from build123d import *

# Parameters (mm, degrees)
EXTRUDE_1_DEPTH                  = 35
SKETCH_2_W                       = 22
SKETCH_2_H                       = 35
EXTRUDE_2_DEPTH                  = 22.75
SKETCH_3_W                       = 11
SKETCH_3_H                       = 15
CUT_EXTRUDE_1_DEPTH              = 32
HOLE_WIZARD_12_5_12_5_1_D        = 12.5
HOLE_WIZARD_12_5_12_5_2_D        = 12.5
HOLE_WIZARD_3_5_3_5_1_D          = 3.5
HOLE_WIZARD_3_5_3_5_1_DEPTH      = 5
SKETCH_10_W                      = 9.5
SKETCH_10_H                      = 18.75
CUT_EXTRUDE_2_DEPTH              = 64.639610362
SKETCH_11_W                      = 22.75
SKETCH_11_H                      = 11
CUT_EXTRUDE_3_DEPTH              = 15
FILLET_2_R                       = 10
SKETCH_13_W                      = 4
SKETCH_13_H                      = 30
EXTRUDE_3_DEPTH                  = 31
SKETCH_16_W                      = 1.75
SKETCH_16_H                      = 4
HOLE_WIZARD_3_5_3_5_2_AT_2_COUNT = 2
HOLE_WIZARD_3_5_3_5_2_AT_2_PITCH = 24
HOLE_WIZARD_3_5_3_5_2_AT_3_COUNT = 2
HOLE_WIZARD_3_5_3_5_2_AT_3_PITCH = 33.941125497
HOLE_WIZARD_3_5_3_5_2_AT_4_COUNT = 2
HOLE_WIZARD_3_5_3_5_2_AT_4_PITCH = 24
SKETCH_17_R                      = 14
CUT_EXTRUDE_4_DEPTH              = 76.494728698
SKETCH_19_W                      = 4
SKETCH_19_H                      = 30
EXTRUDE_5_DEPTH                  = 34
SKETCH_20_R                      = 14
CUT_EXTRUDE_5_DEPTH              = 76.494728698
SKETCH_22_W                      = 1.75
SKETCH_22_H                      = 4
HOLE_WIZARD_3_5_3_5_3_AT_2_COUNT = 2
HOLE_WIZARD_3_5_3_5_3_AT_2_PITCH = 24
HOLE_WIZARD_3_5_3_5_3_AT_3_COUNT = 2
HOLE_WIZARD_3_5_3_5_3_AT_3_PITCH = 33.941125497
HOLE_WIZARD_3_5_3_5_3_AT_4_COUNT = 2
HOLE_WIZARD_3_5_3_5_3_AT_4_PITCH = 24
EXTRUDE_6_DEPTH                  = 4
EXTRUDE_7_DEPTH                  = 4
SKETCH_26_W                      = 10
SKETCH_26_H                      = 4
EXTRUDE_8_DEPTH                  = 35
HOLE_WIZARD_3_5_3_5_4_D          = 3.5
FILLET_7_R                       = 2
FILLET_9_R                       = 5
FILLET_10_R                      = 10
FILLET_12_R                      = 10
FILLET_13_R                      = 2
FILLET_14_R                      = 2
CUT_EXTRUDE_6_DEPTH              = 86.007352664
CUT_EXTRUDE_7_DEPTH              = 15
FILLET_15_R                      = 10


# Some blends are built 0.0001 mm under size
with BuildPart() as part:
    # Sketch 1 → Extrude 1 (new body)
    with BuildSketch(Plane(origin=(0, 35, 0), x_dir=(1, 0, 0), z_dir=(0, 1, 0))):
        with BuildLine():
            Line((35, 0), (13, 0))
            Line((13, 0), (13, -28))
            ThreePointArc((13, -28), (16.514718626, -36.485281374), (25, -40))
            ThreePointArc((25, -40), (32.16515139, -35.913807126), (35, -28.167840434))
            Line((35, -28.167840434), (35, 0))
        make_face()
    extrude(amount=-EXTRUDE_1_DEPTH)

    # Sketch 2 → Extrude 2 (add)
    with BuildSketch(Plane.ZY.offset(-13)):
        with Locations((11, 17.5)):
            Rectangle(SKETCH_2_W, SKETCH_2_H)
    extrude(amount=EXTRUDE_2_DEPTH)

    # Sketch 3 → Cut-Extrude 1 (cut)
    with BuildSketch(Plane.ZY.offset(9.75)):
        with Locations((5.5, 7.5)):
            Rectangle(SKETCH_3_W, SKETCH_3_H)
    extrude(amount=-CUT_EXTRUDE_1_DEPTH, mode=Mode.SUBTRACT)

    # Hole Wizard 12.5 _12.5_1 (through all)
    with Locations(Plane(origin=(0, 35, 0), x_dir=(1, 0, 0), z_dir=(0, 1, 0))):
        with Locations((24, -29)):
            Hole(HOLE_WIZARD_12_5_12_5_1_D / 2)

    # Hole Wizard 12.5 _12.5_2 (through all)
    with Locations(Plane(origin=(35, 0, 0), x_dir=(0, 0, -1), z_dir=(1, 0, 0))):
        with Locations((-11, 25)):
            Hole(HOLE_WIZARD_12_5_12_5_2_D / 2)

    # Hole Wizard 3.5 _3.5_1
    with Locations(Plane(origin=(0, 15, 0), x_dir=(-1, 0, 0), z_dir=(0, -1, 0))):
        with Locations((-17.25, -7), (6.75, -7), (-12.25, -7), (1.75, -7)):
            Hole(HOLE_WIZARD_3_5_3_5_1_D / 2, depth=HOLE_WIZARD_3_5_3_5_1_DEPTH)

    # Sketch 10 → Cut-Extrude 2 (cut, through all)
    with BuildSketch(Plane.XZ):
        with Locations((30.25, 9.375)):
            Rectangle(SKETCH_10_W, SKETCH_10_H)
    extrude(amount=-CUT_EXTRUDE_2_DEPTH, mode=Mode.SUBTRACT)

    # Sketch 11 → Cut-Extrude 3 (cut)
    with BuildSketch(Plane.XZ):
        with Locations((1.625, 16.5)):
            Rectangle(SKETCH_11_W, SKETCH_11_H)
    extrude(amount=-CUT_EXTRUDE_3_DEPTH, mode=Mode.SUBTRACT)

    # Fillet 2
    fillet_2_edges = [part.edges().sort_by_distance(p)[0] for p in [
        (25, 17.5, 40),
    ]]
    fillet(fillet_2_edges, radius=FILLET_2_R)

    # Sketch 19 → Extrude 5 (add)
    with BuildSketch(Plane.ZY.offset(9.75)):
        with Locations((2, 7.5)):
            Rectangle(SKETCH_19_W, SKETCH_19_H)
    extrude(amount=EXTRUDE_5_DEPTH)

    # Sketch 20 → Cut-Extrude 5 (cut, through all)
    with BuildSketch(Plane.XY.offset(4)):
        with Locations((-28.75, 7.5)):
            Circle(SKETCH_20_R)
    extrude(amount=-CUT_EXTRUDE_5_DEPTH, mode=Mode.SUBTRACT)

    # Sketch 22 → Hole Wizard 3.5 _3.5_3 (revolve, cut)
    with BuildSketch(Plane(origin=(-16.75, 19.5, 4), x_dir=(0, -1, 0), z_dir=(1, 0, 0))):
        with Locations((0.875, 2)):
            Rectangle(SKETCH_22_W, SKETCH_22_H)
    hole_wizard_3_5_3_5_3 = revolve(axis=Axis((-16.75, 19.5, 10.35), (0, 0, -1)), mode=Mode.SUBTRACT)

    # Hole Wizard 3.5 _3.5_3 at 2: Hole Wizard 3.5 _3.5_3 ×2
    with Locations(*[(0, -i * HOLE_WIZARD_3_5_3_5_3_AT_2_PITCH, 0) for i in range(1, HOLE_WIZARD_3_5_3_5_3_AT_2_COUNT)]):
        add(hole_wizard_3_5_3_5_3, mode=Mode.SUBTRACT)

    # Hole Wizard 3.5 _3.5_3 at 3: Hole Wizard 3.5 _3.5_3 ×2
    with Locations(*[Vector(-0.7071067811865475, -0.7071067811865476, 0) * (i * HOLE_WIZARD_3_5_3_5_3_AT_3_PITCH) for i in range(1, HOLE_WIZARD_3_5_3_5_3_AT_3_COUNT)]):
        add(hole_wizard_3_5_3_5_3, mode=Mode.SUBTRACT)

    # Hole Wizard 3.5 _3.5_3 at 4: Hole Wizard 3.5 _3.5_3 ×2
    with Locations(*[(-i * HOLE_WIZARD_3_5_3_5_3_AT_4_PITCH, 0, 0) for i in range(1, HOLE_WIZARD_3_5_3_5_3_AT_4_COUNT)]):
        add(hole_wizard_3_5_3_5_3, mode=Mode.SUBTRACT)

    # Sketch 24 → Extrude 6 (add)
    with BuildSketch(Plane.XY.offset(4)):
        Polygon((-9.75, 30.5), (-17.75, 22.5), (-9.75, 22.5), align=None)
    extrude(amount=-EXTRUDE_6_DEPTH)



with BuildPart() as body_2:
    # Sketch 13 → Extrude 3 (new body)
    with BuildSketch(Plane(origin=(25.5, 0, 0), x_dir=(0, 0, -1), z_dir=(1, 0, 0))):
        with Locations((-2, 7.5)):
            Rectangle(SKETCH_13_W, SKETCH_13_H)
    extrude(amount=EXTRUDE_3_DEPTH)

    # Sketch 16 → Hole Wizard 3.5 _3.5_2 (revolve, cut)
    with BuildSketch(Plane(origin=(29.5, -4.5, 4), x_dir=(0, -1, 0), z_dir=(1, 0, 0))):
        with Locations((0.875, 2)):
            Rectangle(SKETCH_16_W, SKETCH_16_H)
    hole_wizard_3_5_3_5_2 = revolve(axis=Axis((29.5, -4.5, 10.35), (0, 0, -1)), mode=Mode.SUBTRACT)

    # Hole Wizard 3.5 _3.5_2 at 2: Hole Wizard 3.5 _3.5_2 ×2
    with Locations(*[(0, i * HOLE_WIZARD_3_5_3_5_2_AT_2_PITCH, 0) for i in range(1, HOLE_WIZARD_3_5_3_5_2_AT_2_COUNT)]):
        add(hole_wizard_3_5_3_5_2, mode=Mode.SUBTRACT)

    # Hole Wizard 3.5 _3.5_2 at 3: Hole Wizard 3.5 _3.5_2 ×2
    with Locations(*[Vector(0.7071067811865475, 0.7071067811865476, 0) * (i * HOLE_WIZARD_3_5_3_5_2_AT_3_PITCH) for i in range(1, HOLE_WIZARD_3_5_3_5_2_AT_3_COUNT)]):
        add(hole_wizard_3_5_3_5_2, mode=Mode.SUBTRACT)

    # Hole Wizard 3.5 _3.5_2 at 4: Hole Wizard 3.5 _3.5_2 ×2
    with Locations(*[(i * HOLE_WIZARD_3_5_3_5_2_AT_4_PITCH, 0, 0) for i in range(1, HOLE_WIZARD_3_5_3_5_2_AT_4_COUNT)]):
        add(hole_wizard_3_5_3_5_2, mode=Mode.SUBTRACT)

    # Sketch 17 → Cut-Extrude 4 (cut, through all)
    with BuildSketch(Plane.XY.offset(4)):
        with Locations((41.5, 7.5)):
            Circle(SKETCH_17_R)
    extrude(amount=-CUT_EXTRUDE_4_DEPTH, mode=Mode.SUBTRACT)


with BuildPart() as part_1:
    add(part.part)

    add(body_2.part)  # Extrude 7 merges body 2
    # Sketch 25 → Extrude 7 (add)
    with BuildSketch(Plane.XY.offset(4)):
        Polygon((33.5, 22.5), (25.5, 30.5), (25.5, 22.5), align=None)
    extrude(amount=-EXTRUDE_7_DEPTH)

    # Sketch 26 → Extrude 8 (add)
    with BuildSketch(Plane.XY.offset(22)):
        with Locations((5.25, 17)):
            Rectangle(SKETCH_26_W, SKETCH_26_H)
    extrude(amount=EXTRUDE_8_DEPTH)

    # Hole Wizard 3.5 _3.5_4 (through all)
    with Locations(Plane(origin=(0, 15, 0), x_dir=(-1, 0, 0), z_dir=(0, -1, 0))):
        with Locations((-5.25, -52), (-5.25, -42), (-5.25, -32)):
            Hole(HOLE_WIZARD_3_5_3_5_4_D / 2)

    # Fillet 7
    fillet_7_edges = [part_1.edges().sort_by_distance(p)[0] for p in [
        (0.25, 17, 22),
        (10.25, 17, 22),
    ]]
    fillet(fillet_7_edges, radius=FILLET_7_R)

    # Fillet 9
    fillet_9_edges = [part_1.edges().sort_by_distance(p)[0] for p in [
        (0.25, 17, 57),
        (10.25, 17, 57),
    ]]
    fillet(fillet_9_edges, radius=FILLET_9_R - 0.0001)  # a hair under: the kernel refuses the full size

    # Fillet 10
    # the kernel refuses this fillet: 10 mm, written as the material it takes off along each edge
    with BuildSketch(Plane(origin=(35, -32.046488893, 18.75), x_dir=(-0.03816406367220006, 0, 0.999271486756239), z_dir=(0, 1, 0))) as fillet_10_piece_1:
        with BuildLine():
            CenterArc((10.360556073, -9.693195649), FILLET_10_R, 75.770650452, 103.082689776)
            Line((0.362558605, -9.493079124), (-0.637241142, -9.473067472))
            ThreePointArc((-0.637241142, -9.473067472), (-0.817992184, -4.784703626), (-0.999271487, -0.038164064))
            Line((-0.999271487, -0.038164064), (-0.038164064, 0.999271487))
            ThreePointArc((-0.038164064, 0.999271487), (9.372815349, 1.358694549), (13.064399506, 0.969319565))
            Line((13.064399506, 0.969319565), (12.818595557, 0))
        make_face()
    extrude(amount=99.092977786, mode=Mode.SUBTRACT)

    # Fillet 12
    fillet_12_edges = [part_1.edges().sort_by_distance(p)[0] for p in [
        (1.625, 35, 22),
    ]]
    fillet(fillet_12_edges, radius=FILLET_12_R)

    # Fillet 13
    fillet_13_edges = [part_1.edges().sort_by_distance(p)[0] for p in [
        (-9.75, 30.5, 2),
        (-9.75, -7.5, 2),
        (-43.75, 22.5, 2),
        (-43.75, -7.5, 2),
        (-17.75, 22.5, 2),
    ]]
    fillet(fillet_13_edges, radius=FILLET_13_R)

    # Fillet 14
    fillet_14_edges = [part_1.edges().sort_by_distance(p)[0] for p in [
        (56.5, 22.5, 2),
        (25.5, 30.5, 2),
        (33.5, 22.5, 2),
        (25.5, -7.5, 2),
        (56.5, -7.5, 2),
    ]]
    fillet(fillet_14_edges, radius=FILLET_14_R)

    # Sketch 32 → Cut-Extrude 6 (cut, through all)
    with BuildSketch(Plane.XY.offset(4)):
        with BuildLine():
            Line((-9.75, 2.270340952), (-9.75, 15))
            ThreePointArc((-9.75, 15), (-10.952290213, 8.635170476), (-9.75, 2.270340952))
        make_face()
    extrude(amount=-CUT_EXTRUDE_6_DEPTH, mode=Mode.SUBTRACT)

    # Sketch 33 → Cut-Extrude 7 (cut)
    with BuildSketch(Plane.XZ):
        with BuildLine():
            Line((13, 22), (13, 11))
            Line((13, 11), (22.25, 11))
            ThreePointArc((22.25, 11), (19.219835157, 17.841111382), (13, 22))
        make_face()
    extrude(amount=-CUT_EXTRUDE_7_DEPTH, mode=Mode.SUBTRACT)

    # Fillet 15
    fillet_15_edges = [part_1.edges().sort_by_distance(p)[0] for p in [
        (13, 7.5, 22),
    ]]
    fillet(fillet_15_edges, radius=FILLET_15_R)


solid = part_1.part
Can you work these out from the model? Positions are in its coordinate system, mm. A direction names the side the tool comes from. Round coordinates to 2 decimals unless told otherwise and drop trailing zeros. Write each loop counter-clockwise with the first axis right and the second up, starting at its lowest first coordinate (ties: lowest second). Pieces come first, ordered by that corner, then holes. Notation, with made-up numbers: M 20,-13.5 L 44,-13.5 A13 cw 44,-6.5 Z; hole C 86.5,34 d8. An arc over 180 degrees is marked long. Use a Markdown table: item, result.
Item 1: I want a section at A-A (z = 42). List the corners of the cut face in (x, y) for me.
Found:
| item | result |
|---|---|
| outline | M 0.25,15 L 3.5,15 L 3.5,19 L 0.25,19 Z; M 7,15 L 10.25,15 L 10.25,19 L 7,19 Z |
Item 2: For pin 1 Ø5.5 at (x, y) = (-40.75, 19.5) entering from +Z; pin 2 Ø17 at (x, y) = (-28.75, 7.5) entering from +Z; pin 3 Ø0.6 at (x, z) = (-1, 6) entering from -Y; pin 4 Ø6 at (y, z) = (16.5, 36.5) entering from -X, each with a flat end and sliding along its axis, tell me the tip position at first contact or that it passes through.
Found:
| item | result |
|---|---|
| pin 1 | stops at z = 4 |
| pin 2 | passes through |
| pin 3 | stops at y = 20 |
| pin 4 | stops at x = 0.25 |
Item 3: I want a section at B-B (x = 41.5). List the corners of the cut face in (y, z) for me.
Found:
| item | result |
|---|---|
| outline | M -7.5,0 L -6.5,0 L -6.5,4 L -7.5,4 Z; M 21.5,0 L 22.5,0 L 22.5,4 L 21.5,4 Z |
Item 4: Which directions (+Z, -Z, +X, -X, +Y, -Y) give clear straight access to the entire face, cutting with the end or side of a thin tool? Please do faces 1 (the face through (6, 15, 22)), 2 (the face through (0.25, 17, 38)), 3 (the face through (-9.75, -2, 2)).
Found:
| item | result |
|---|---|
| face 1 | -Z, -Y |
| face 2 | +Z, -X, +Y, -Y |
| face 3 | +Z, -Z, -Y |
Item 5: I want a section at C-C (y = -4.5). State how many separate pieces and enclosed holes the cut face has, and give its area (3 significant figures).
Found:
| item | result |
|---|---|
| separate pieces | 8 |
| enclosed holes | 0 |
| area | 88.6 mm2 |
Item 6: We'd pull the mould along X, two halves only. Please class faces 4 (the face through (55.9, -6.93, 1.97)), 5 (the face through (-43.75, 8, 2)), 6 (the face through (10.25, 17, 38)): released by +X, released by -X, zero draft, split by the parting line, or undercut.
Found:
| item | result |
|---|---|
| face 4 | released by +X |
| face 5 | released by -X |
| face 6 | undercut |
Item 7: If I drill on line 1 along X through (y, z) = (17.65, 7); line 2 along Y through (x, z) = (-40.75, 1.5); line 3 along Z through (x, y) = (5.25, 17.8), over which ranges is the centre line in solid material (lowest first)? Write a range as [from, to].
Found:
| item | result |
|---|---|
| line 1 | x = [-9.75, -8.5], [-5, -3.5], [0, 10.5], [14, 15.5], [19, 25.5] |
| line 2 | y = [-7.5, -6.25], [-2.75, 0.29], [14.71, 17.75], [21.25, 22.5] |
| line 3 | z = [0, 30.25], [33.75, 40.25], [43.75, 50.25], [53.75, 57] |
